from build123d import *

# Parameters (mm, degrees)
SKETCH9_W           = 50
SKETCH9_H           = 110
BOSS_EXTRUDE3_DEPTH = 40
CUT_EXTRUDE4_DEPTH  = 90
FILLET2_R           = 20
SKETCH15_R          = 10
CUT_EXTRUDE5_DEPTH  = 41
SKETCH22_R          = 10
BOSS_EXTRUDE4_DEPTH = 20


with BuildPart() as part:
    # Sketch9 → Boss-Extrude3 (new body)
    with BuildSketch(Plane(origin=(-33.280188112, 0, 144.42881153), x_dir=(-0.973697035, 0, -0.227846622), z_dir=(0, 1, 0))):
        with Locations((25.502796398, -93.212684061)):
            Rectangle(SKETCH9_W, SKETCH9_H)
    extrude(amount=-BOSS_EXTRUDE3_DEPTH)

    # Sketch14 → Cut-Extrude4 (cut)
    with BuildSketch(Plane(origin=(1.578968454, -248.415731332, 0.369481077), x_dir=(0.949498442, -0.221555699, 0.222184114), z_dir=(-0.227846622, 0, 0.973697035))):
        Polygon((-102.607181661, 218.615622522), (-99.28384617, 203.988406751), (-50.526460266, 215.066191719), (-53.849795757, 229.69340749), align=None)
    extrude(amount=CUT_EXTRUDE4_DEPTH, mode=Mode.SUBTRACT)

    # Fillet2
    fillet2_edges = [part.edges().sort_by_distance(p)[0] for p in [
        (0, -6.25, 0),
        (-48.684851767, -6.25, -11.392331125),
        (-48.684851767, -33.75, -11.392331125),
        (0, -33.75, 0),
    ]]
    fillet(fillet2_edges, radius=FILLET2_R)

    # Sketch15 → Cut-Extrude5 (cut, through all)
    with BuildSketch(Plane(origin=(0, -40, 0), x_dir=(0.973697035, 0, 0.227846622), z_dir=(0, -1, 0))):
        with Locations((-25, 20)):
            Circle(SKETCH15_R)
    extrude(amount=-CUT_EXTRUDE5_DEPTH, mode=Mode.SUBTRACT)

    # Sketch22 → Boss-Extrude4 (add)
    with BuildSketch(Plane(origin=(-24.856078548, -32.574722266, 107.155123892), x_dir=(-0.94660116, -0.234267522, -0.221506145), z_dir=(-0.227846622, 0, 0.973697035))):
        with Locations((21.565180907, -18.131298438)):
            Circle(SKETCH22_R)
    extrude(amount=BOSS_EXTRUDE4_DEPTH)


solid = part.part
The listing builds one solid part. Answer for the finished solid, in the listing's coordinates (mm). A direction names the side the tool comes from. Round coordinates to 2 decimals unless told otherwise and drop trailing zeros. Loops run counter-clockwise (first coordinate to the right, second up) from the corner with the lowest first, then second, coordinate; pieces in that order, holes last. Notation, with made-up numbers: M 9.25,64.5 L 49.25,64.5 A11 cw 49.25,81.5 Z; hole C 73.25,48 d8. An arc over 180 degrees is marked long. Write each question's results on one line, items separated by ' | '. Start each with the question number.
1) Which of the six approach directions +Z, -Z, +X, -X, +Y, -Y give full straight-line access (tool end or side, diameter ignored) to faces 4 (the flat face through (-14.666, -10.831, 62.677)), 5 (the flat face through (-45.156, -19.744, 81.865))?
2) Each of these flat-tipped pins is pushed along its axis until it touches: pin 1 (2 mm diameter, centred on x = -43, y = -13, fed in from -Z); pin 2 (5 mm diameter, centred on y = -12, z = 34, fed in from +X); pin 3 (3 mm diameter, centred on x = -42, y = -15, fed in from -Z). Where does it stop, or does it pass through?
3) Straight lines are drawn through the part: probe 1 along Y at (x, z) = (-37.5, 76); probe 2 along Z at (x, y) = (-32, -12); probe 3 along Z at (x, y) = (-32.5, -11). For each, find the intervals that lie inside material, in ascending order.
4) Determine the mould class of faces 1 (the flat face through (-37, 0, 49)), 2 (the flat face through (-34, -12.5, 38)), 3 (the flat face through (-63.35, -10.83, 51.28)) for opening direction Y: pulls with the +Y half, pulls with the -Y half, needs draft (parallel to the pull), parting line crosses it, or undercut.
5) Find section C-C on z = 54.5. Write down the section's boundary in (x, y).
6) Find section B-B on y = -33. Write down the section's boundary in (x, z).
7) Find section A-A on z = 14.5. Write down the section's boundary in (x, y), plus the area to 3 significant figures.
8) Find section D-D on y = -14. Write down the section's boundary in (x, z).
Final values:
1) face 4: +Z, +X, +Y, -Y | face 5: -Z, +X
2) pin 1: z = -5.53 | pin 2: x = -7.37 | pin 3: z = 82.25
3) probe 1: -40 to -27.5, -12.5 to 0 | probe 2: -7.28 to 4.27, 23.28 to 105.48 | probe 3: -7.32 to 4.45, 23.11 to 105.37
4) face 1: pulls with the +Y half | face 2: undercut | face 3: needs draft
5) outline: M -64.1,-40 L -12.75,-40 L -12.75,-27.5 L -64.1,-27.5 Z; M -64.1,-12.5 L -12.75,-12.5 L -12.75,0 L -64.1,0 Z
6) outline: M -73.75,95.71 L -53.24,8.08 A20 ccw -29.21,-6.84 L -19.47,-4.56 A20 ccw -4.56,19.47 L -25.06,107.11 Z; hole C -28.9,13.78 d20
7) outline: M -54.74,-40 L -38.87,-40 L -38.87,-27.5 L -54.74,-27.5 Z; M -54.74,-12.5 L -38.87,-12.5 L -38.87,0 L -54.74,0 Z; M -18.93,-40 L -4.04,-40 L -4.04,-27.5 L -18.93,-27.5 Z; M -18.93,-12.5 L -4.04,-12.5 L -4.04,0 L -18.93,0 Z | area: 769 mm²
8) outline: M -73.75,95.71 L -69.19,76.24 L -20.51,87.63 L -25.06,107.11 L -41.62,103.23 L -46.17,122.71 L -61.75,119.06 L -57.2,99.59 Z
